from build123d import *

# Parameters (mm, degrees)
PAD015_DEPTH             = 3
SKETCH096_R              = 1.7
POCKET062_DEPTH          = 2019.841851
POCKET062_DEPTH_BACK     = 2022.841851
POLARPATTERN017_COUNT    = 3
CLONE004_PLACEMENT_ANGLE = 90


with BuildPart() as part:
    # Sketch095 → Pad015 (new body)
    with BuildSketch(Plane.XY):
        with BuildLine():
            ThreePointArc((337.01048, -215.462146), (350.845307, 192.113432), (0, 400))
            Line((0, 330), (0, 400))
            ThreePointArc((276.422258, -180.251866), (290.157816, 157.189192), (0, 330))
            ThreePointArc((276.422258, -180.251866), (276.152366, -181.809361), (277.097544, -183.076353))
            Line((277.097544, -183.076353), (334.325427, -216.116886))
            ThreePointArc((334.325427, -216.116886), (335.799237, -216.327901), (337.01048, -215.462146))
        make_face()
    pad015 = extrude(amount=PAD015_DEPTH)

    # Mirrored026: Pad015 across Sketch095 V_Axis
    add(pad015.mirror(Plane(origin=(0, 0, 0), x_dir=(0, 0, 1), z_dir=(1, 0, 0))))

    # Sketch096 → Pocket062 (cut, two sides)
    with BuildSketch(Plane(origin=(0, 330, 0), x_dir=(1, 0, 0), z_dir=(0, 0, 1))) as pocket062_sk:
        with Locations((0, 10)):
            Circle(SKETCH096_R)
        with Locations((0, 35)):
            Circle(SKETCH096_R)
        with Locations((0, 60)):
            Circle(SKETCH096_R)
    pocket062 = extrude(amount=-POCKET062_DEPTH, mode=Mode.SUBTRACT) + extrude(pocket062_sk.sketch, amount=POCKET062_DEPTH_BACK, mode=Mode.SUBTRACT)

    # PolarPattern017: Pocket062 ×3 about axis
    polarpattern017_axis = Axis((0, 0, 0), (0, 0, 1))
    for i in range(1, POLARPATTERN017_COUNT):
        add(pocket062.rotate(polarpattern017_axis, i * 360 / POLARPATTERN017_COUNT), mode=Mode.SUBTRACT)


with BuildPart() as part_1:
    # Clone004 placement: moved
    add(part.part.moved(Location((-216.377145, 400, 0))).rotate(Axis((-216.377145, 400, 0), (0, 0, 1)), CLONE004_PLACEMENT_ANGLE))


solid = part_1.part
Build history of the part. All positions in model axes, mm. A direction names the side the tool comes from. Round coordinates to 2 decimals unless told otherwise and drop trailing zeros. Loops run counter-clockwise (first coordinate to the right, second up) from the corner with the lowest first, then second, coordinate; pieces in that order, holes last. Notation, with made-up numbers: (22, 64.25) -> (36, 64.25) arc R17 cw to (36, 81.25) -> close; hole circle Ø11 at (60, 78.25). An arc over 180 degrees is marked (long way). One line per item, written item: value. Start each with the question number.
Q1. Probe line 1 along Y through (x, z) = (-163.5, 2.15); line 2 along Y through (x, z) = (-365.5, 1.35); line 3 along X through (y, z) = (393, 1.4). List the from-to ranges inside material, lowest first.
Q2. Cut at B-B on z = 1.6. Count the separate pieces of the cut face and the enclosed holes in it, plus the area to 3 significant figures.
Q3. Cut at D-D on y = 513.5. List the corners of the cut face in (x, z), plus the area to 3 significant figures.
Q4. Drop a flat-ended pin along its axis: pin 1 Ø1 at (y, z) = (525.5, 0.5) entering from -X. Give the stop position or say it passes through.
Q5. Cut at C-C on x = -417. List the corners of the cut face in (y, z).
Q6. Two-plate mould, pull along Y, no slides. Class faces 3 (the face through (-538, 313, 0)), 4 (the face through (-17.012, 705.311, 1.479)): released by +Y, released by -Y, zero draft, split by the parting line, or undercut.
Q7. 3-axis set-ups, long thin cutter, end or side, ignore diameter. For faces 1 (the face through (-538, 313, 3)), 2 (the face through (-17.012, 94.689, 1.479)): which of +Z, -Z, +X, -X, +Y, -Y reach the whole face in a straight line?
Q8. Cut at A-A on x = -324.5. List the corners of the cut face in (y, z), plus the area to 3 significant figures.
Computed:
1. line 1: 3.51 to 74.26, 725.74 to 796.49
1. line 2: 28.84 to 105.62, 694.38 to 771.16
1. line 3: -616.32 to -546.3
2. separate pieces: 1
2. enclosed holes: 9
2. area: 110,000 mm²
3. outline: (-599.94, 0) -> (-526.24, 0) -> (-526.24, 3) -> (-599.94, 3) -> close
3. area: 221 mm²
4. pin 1: x = -596.34
5. outline: (53.95, 0) -> (137.99, 0) -> (137.99, 3) -> (53.95, 3) -> close; (662.01, 0) -> (746.05, 0) -> (746.05, 3) -> (662.01, 3) -> close
6. face 3: zero draft
6. face 4: undercut
7. face 1: +Z, +X, -X, +Y, -Y
7. face 2: +Z, -Z, +X
8. outline: (14.89, 0) -> (88.22, 0) -> (88.22, 3) -> (14.89, 3) -> close; (711.78, 0) -> (785.11, 0) -> (785.11, 3) -> (711.78, 3) -> close
8. area: 440 mm²
